Read the model definition and answer for the solid it produces. Units are mm, in the model's axes. Face numbers are marked on the shaded views. Coordinates: 2 decimals unless noted, no trailing zeros. Write each loop counter-clockwise with the first axis right and the second up, starting at its lowest first coordinate (ties: lowest second). Pieces come first, ordered by that corner, then holes.
1) The part is cut by section D-D (x = 13.97). Determine the outline of the cut face in (y, z).
2) Determine the mould class of the marked faces 1 and 2 for opening direction X: +X half, -X half, draft (parallel to the pull), parting line (faces both ways), or undercut.
3) The part is cut by section A-A (x = 0). Determine the outline of the cut face in (y, z) (3 decimals).
4) Each of these flat-tipped pins is pushed along its axis until it touches: pin 1 Ø1.5 at (x, z) = (8.495, 0) entering from -Y; pin 2 Ø1.5 at (y, z) = (1, -1.5) entering from +X; pin 3 Ø2 at (x, y) = (-12, -0.5) entering from +Z. Where does it stop, or does it pass through?
5) The part is cut by section C-C (y = -2.1). Determine the outline of the cut face in (x, z).
6) The part is cut by section B-B (z = 0). Give the number of separate pieces and of enclosed holes in the cut face, then the cut area to 3 significant figures.
7) Find the intervals of material crossed by line 1 (X direction, y = 1.2, z = 1.5); line 2 (Y direction, x = -4.5, z = 2.25); line 3 (Z direction, x = 13.97, y = 0.95), in increasing order.
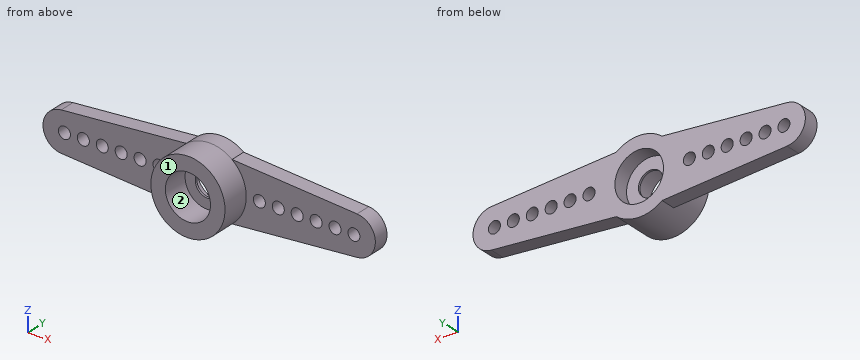
from build123d import *

# Parameters (mm, degrees)
SKETCH1_R               = 2.345
EXTRUDE1_DEPTH          = 1.5
SKETCH2_R               = 3.58
SKETCH2_R_2             = 2.18
EXTRUDE2_DEPTH          = 2.74
SKETCH3_R               = 2.345
SKETCH3_R_2             = 1.195
EXTRUDE3_DEPTH          = 0.2
SKETCH4_R               = 0.58
EXTRUDE4_DEPTH          = 5.24
LPATTERN1_COUNT         = 6
LPATTERN1_PITCH         = 1.825
MIRROR1_COPY_1_SKETCH_R = 0.58
MIRROR1_COPY_1_DEPTH    = 5.24
MIRROR1_COPY_2_SKETCH_R = 0.58
MIRROR1_COPY_2_DEPTH    = 5.24
MIRROR1_COPY_3_SKETCH_R = 0.58
MIRROR1_COPY_3_DEPTH    = 5.24
MIRROR1_COPY_4_SKETCH_R = 0.58
MIRROR1_COPY_4_DEPTH    = 5.24
MIRROR1_COPY_5_SKETCH_R = 0.58
MIRROR1_COPY_5_DEPTH    = 5.24


with BuildPart() as part:
    # Sketch1 → Extrude1 (new body)
    with BuildSketch(Plane(origin=(0, 0, 0), x_dir=(1, 0, 0), z_dir=(0, 1, 0))):
        with BuildLine():
            Line((-14.274464235, -1.904528835), (-2.2054478, -2.82))
            ThreePointArc((-2.2054478, -2.82), (0, -3.58), (2.2054478, -2.82))
            Line((2.2054478, -2.82), (14.274464235, -1.904528835))
            ThreePointArc((14.274464235, -1.904528835), (16.04, 0), (14.274464235, 1.904528835))
            Line((14.274464235, 1.904528835), (2.2054478, 2.82))
            ThreePointArc((2.2054478, 2.82), (0, 3.58), (-2.2054478, 2.82))
            Line((-2.2054478, 2.82), (-14.274464235, 1.904528835))
            ThreePointArc((-14.274464235, 1.904528835), (-16.04, 0), (-14.274464235, -1.904528835))
        make_face()
        with Locations(Location((0, 0, 0), (0, 0, 270))):  # turned: the seam where the file's is
            Circle(SKETCH1_R, mode=Mode.SUBTRACT)
    extrude(amount=EXTRUDE1_DEPTH)

    # Sketch2 → Extrude2 (add)
    with BuildSketch(Plane.XZ):
        with Locations(Location((0, 0, 0), (0, 0, 270))):  # turned: the seam where the file's is
            Circle(SKETCH2_R)
        with Locations(Location((0, 0, 0), (0, 0, 270))):  # turned: the seam where the file's is
            Circle(SKETCH2_R_2, mode=Mode.SUBTRACT)
    extrude(amount=EXTRUDE2_DEPTH)

    # Sketch3 → Extrude3 (add)
    with BuildSketch(Plane(origin=(0, 0, 0), x_dir=(-1, 0, 0), z_dir=(0, 1, 0))):
        with Locations(Location((0, 0, 0), (0, 0, 90))):  # turned: the seam where the file's is
            Circle(SKETCH3_R)
        with Locations(Location((0, 0, 0), (0, 0, 90))):  # turned: the seam where the file's is
            Circle(SKETCH3_R_2, mode=Mode.SUBTRACT)
    extrude(amount=-EXTRUDE3_DEPTH)

    # Sketch4 → Extrude4 (cut, through all)
    with BuildSketch(Plane(origin=(0, 1.5, 0), x_dir=(1, 0, 0), z_dir=(0, 1, 0))):
        with Locations(Location((-4.845, 0, 0), (0, 0, 270))):  # turned: the seam where the file's is
            Circle(SKETCH4_R)
    extrude4 = extrude(amount=-EXTRUDE4_DEPTH, mode=Mode.SUBTRACT)

    # LPattern1: Extrude4 ×6
    with Locations(*[(-i * LPATTERN1_PITCH, 0, 0) for i in range(1, LPATTERN1_COUNT)]):
        add(extrude4, mode=Mode.SUBTRACT)

    # Mirror1: Extrude4 across plane
    add(extrude4.mirror(Plane(origin=(0, 0, 0), x_dir=(0, 0, 1), z_dir=(1, 0, 0))), mode=Mode.SUBTRACT)

    # Mirror1 copy 1 sketch → Mirror1 copy 1 (cut, through all)
    with BuildSketch(Plane(origin=(1.825, 1.5, 0), x_dir=(-1, 0, 0), z_dir=(0, 1, 0))):
        with Locations((-4.845, 0)):
            Circle(MIRROR1_COPY_1_SKETCH_R)
    extrude(amount=-MIRROR1_COPY_1_DEPTH, mode=Mode.SUBTRACT)

    # Mirror1 copy 2 sketch → Mirror1 copy 2 (cut, through all)
    with BuildSketch(Plane(origin=(3.65, 1.5, 0), x_dir=(-1, 0, 0), z_dir=(0, 1, 0))):
        with Locations((-4.845, 0)):
            Circle(MIRROR1_COPY_2_SKETCH_R)
    extrude(amount=-MIRROR1_COPY_2_DEPTH, mode=Mode.SUBTRACT)

    # Mirror1 copy 3 sketch → Mirror1 copy 3 (cut, through all)
    with BuildSketch(Plane(origin=(5.475, 1.5, 0), x_dir=(-1, 0, 0), z_dir=(0, 1, 0))):
        with Locations((-4.845, 0)):
            Circle(MIRROR1_COPY_3_SKETCH_R)
    extrude(amount=-MIRROR1_COPY_3_DEPTH, mode=Mode.SUBTRACT)

    # Mirror1 copy 4 sketch → Mirror1 copy 4 (cut, through all)
    with BuildSketch(Plane(origin=(7.3, 1.5, 0), x_dir=(-1, 0, 0), z_dir=(0, 1, 0))):
        with Locations((-4.845, 0)):
            Circle(MIRROR1_COPY_4_SKETCH_R)
    extrude(amount=-MIRROR1_COPY_4_DEPTH, mode=Mode.SUBTRACT)

    # Mirror1 copy 5 sketch → Mirror1 copy 5 (cut, through all)
    with BuildSketch(Plane(origin=(9.125, 1.5, 0), x_dir=(-1, 0, 0), z_dir=(0, 1, 0))):
        with Locations((-4.845, 0)):
            Circle(MIRROR1_COPY_5_SKETCH_R)
    extrude(amount=-MIRROR1_COPY_5_DEPTH, mode=Mode.SUBTRACT)


solid = part.part
Reported:
1. outline: (0, -1.93) - (1.5, -1.93) - (1.5, -0.58) - (0, -0.58) - close; (0, 0.58) - (1.5, 0.58) - (1.5, 1.93) - (0, 1.93) - close
2. face 1: draft
2. face 2: undercut
3. outline: (-2.74, -3.58) - (1.5, -3.58) - (1.5, -2.345) - (0, -2.345) - (0, -1.195) - (-0.2, -1.195) - (-0.2, -2.18) - (-2.74, -2.18) - close; (-2.74, 2.18) - (-0.2, 2.18) - (-0.2, 1.195) - (0, 1.195) - (0, 2.345) - (1.5, 2.345) - (1.5, 3.58) - (-2.74, 3.58) - close
4. pin 1: stops at y = 0
4. pin 2: stops at x = 15.89
4. pin 3: stops at z = 2.14
5. outline: circle Ø7.16 at (0, 0); hole circle Ø4.36 at (0, 0)
6. separate pieces: 14
6. enclosed holes: 0
6. area: 28.3 mm2
7. line 1: x = -15.31 to -1.8, 1.8 to 15.31
7. line 2: y = 0 to 1.5
7. line 3: z = -1.93 to -0.58, 0.58 to 1.93
